```python
from build123d import *

# Parameters (mm, degrees)
SKETCH_1_W          = 125
SKETCH_1_H          = 40
SKETCH_1_R          = 1.6
SKETCH_1_W_2        = 45
SKETCH_1_H_2        = 3
EXTRUDE_1_DEPTH     = 2
SKETCH_2_W          = 4
SKETCH_2_H          = 40
CUT_EXTRUDE_1_DEPTH = 10
FILLET_1_R          = 3
FILLET_2_R          = 1


with BuildPart() as part:
    # 草图1 → 凸台-拉伸1 (new body)
    # profile 1 of 3: a face of its own
    with BuildSketch(Plane(origin=(0, 0, 0), x_dir=(1, 0, 0), z_dir=(0, 1, 0))):
        Rectangle(SKETCH_1_W, SKETCH_1_H)
        with Locations(Location((60, 16, 0), (0, 0, 270))):
            Circle(SKETCH_1_R, mode=Mode.SUBTRACT)
        with Locations(Location((60, 5, 0), (0, 0, 270))):
            Circle(SKETCH_1_R, mode=Mode.SUBTRACT)
        with Locations(Location((60, -5, 0), (0, 0, 270))):
            Circle(SKETCH_1_R, mode=Mode.SUBTRACT)
        with Locations(Location((60, -16, 0), (0, 0, 270))):
            Circle(SKETCH_1_R, mode=Mode.SUBTRACT)
        with BuildLine():
            Line((-50.5, -2.5), (50.5, -2.5))
            ThreePointArc((50.5, -2.5), (51.914213562, -1.914213562), (52.5, -0.5))
            Line((52.5, -0.5), (52.5, 0.5))
            ThreePointArc((52.5, 0.5), (51.914213562, 1.914213562), (50.5, 2.5))
            Line((50.5, 2.5), (-50.5, 2.5))
            ThreePointArc((-50.5, 2.5), (-51.914213562, 1.914213562), (-52.5, 0.5))
            Line((-52.5, 0.5), (-52.5, -0.5))
            ThreePointArc((-52.5, -0.5), (-51.914213562, -1.914213562), (-50.5, -2.5))
        make_face(mode=Mode.SUBTRACT)
    # profile 2 of 3: a face of its own
    with BuildSketch(Plane(origin=(0, 0, 0), x_dir=(1, 0, 0), z_dir=(0, 1, 0))):
        with Locations((-30, -21.5)):
            Rectangle(SKETCH_1_W_2, SKETCH_1_H_2)
    # profile 3 of 3: a face of its own
    with BuildSketch(Plane(origin=(0, 0, 0), x_dir=(1, 0, 0), z_dir=(0, 1, 0))):
        with Locations((-30, 21.5)):
            Rectangle(SKETCH_1_W_2, SKETCH_1_H_2)
    extrude(amount=EXTRUDE_1_DEPTH)

    # 草图2 → 切除-拉伸1 (cut)
    with BuildSketch(Plane(origin=(0, 2, 0), x_dir=(1, 0, 0), z_dir=(0, 1, 0))):
        with Locations((-60.5, 0)):
            Rectangle(SKETCH_2_W, SKETCH_2_H)
    extrude(amount=-CUT_EXTRUDE_1_DEPTH, mode=Mode.SUBTRACT)

    # 圆角1
    fillet_1_edges = [part.edges().sort_by_distance(p)[0] for p in [
        (62.5, 1, -20),
        (62.5, 1, 20),
        (-58.5, 1, -20),
        (-58.5, 1, 20),
    ]]
    fillet(fillet_1_edges, radius=FILLET_1_R)

    # 圆角2
    fillet_2_edges = [part.edges().sort_by_distance(p)[0] for p in [
        (-52.5, 1, -23),
        (-7.5, 1, -23),
        (-7.5, 1, 23),
        (-52.5, 1, 23),
    ]]
    fillet(fillet_2_edges, radius=FILLET_2_R)


solid = part.part
```
Model file for the job. Use its own axes, mm. A direction names the side the tool comes from. Give positions to 0.01 mm unless a question says otherwise; leave off trailing zeros. Order: outer loops, then holes, each group sorted by start corner. A loop starts at its lowest first (then second) coordinate and runs counter-clockwise, first axis right, second up.
1) Saw through at C-C, the plane y = 1. Count the separate pieces of the cut face and the enclosed holes in it, then the cut area to 3 significant figures.
2) Saw through at B-B, the plane z = -5. Write the cut outline in (x, y).
3) Pin check, flat tips, straight feed: pin 1 (1 mm diameter, centred on x = 49.5, y = 1.5, fed in from -Z); pin 2 (1 mm diameter, centred on x = 34.5, z = 1.5, fed in from -Y); pin 3 (0.6 mm diameter, centred on x = 41, y = 0.5, fed in from +Z); pin 4 (0.6 mm diameter, centred on y = 1, z = 20.5, fed in from +X). Stop position of each tip, or through.
4) Saw through at A-A, the plane x = 0.5. Write the cut outline in (y, z), then the cut area to 3 significant figures.
5) 3-axis set-ups, long thin cutter, end or side, ignore diameter. For faces 1 (the flat face through (1, 2, -5)), 2 (the flat face through (-52.5, 1, 21)), 3 (the flat face through (-54, 1, -20)), 4 (the flat face through (-1, 1, 2.5)), 5 (the flat face through (26, 1, -20)): which of +Z, -Z, +X, -X, +Y, -Y reach the whole face in a straight line?
6) Mould opens along X. For faces 6 (the cylindrical face through (-51.9, 0.99, -1.93)), 7 (the flat face through (-7.5, 1, 21)), 8 (the flat face through (26, 1, 20)) say: +X half, -X half, draft (parallel to the pull), parting line (faces both ways), or undercut.
7) Wall check: probe 1 along X at (y, z) = (1.35, -16); probe 2 along Z at (x, y) = (-18.5, 0.2); probe 3 along X at (y, z) = (0.5, -0.5). Give the ranges that are in metal, low to high.
Computed:
1. separate pieces: 1
1. enclosed holes: 5
1. area: 4,550 mm2
2. outline: (-58.5, 0) - (58.4, 0) - (58.4, 2) - (-58.5, 2) - close; (61.6, 0) - (62.5, 0) - (62.5, 2) - (61.6, 2) - close
3. pin 1: stops at z = -20
3. pin 2: passes through
3. pin 3: stops at z = 20
3. pin 4: stops at x = -7.5
4. outline: (0, -20) - (2, -20) - (2, -2.5) - (0, -2.5) - close; (0, 2.5) - (2, 2.5) - (2, 20) - (0, 20) - close
4. area: 70.0 mm2
5. face 1: +Z, -Z, +X, -X, +Y
5. face 2: +Z, -X, +Y, -Y
5. face 3: -Z, -X, +Y, -Y
5. face 4: +Y, -Y
5. face 5: -Z, +X, +Y, -Y
6. face 6: undercut
6. face 7: +X half
6. face 8: draft
7. probe 1: x = -58.5 to 58.4, 61.6 to 62.5
7. probe 2: z = -23 to -2.5, 2.5 to 23
7. probe 3: x = -58.5 to -52.5, 52.5 to 62.5
